Autodesk Inventor part; units mm, degrees
ref_plane "YZ Plane" through (0, 0, 0) normal (1, 0, 0) x (0, 1, 0)
ref_plane "XZ Plane" through (0, 0, 0) normal (0, 1, 0) x (-1, 0, 0)
ref_plane "XY Plane" through (0, 0, 0) normal (0, 0, 1) x (1, 0, 0)
sketch "Sketch1" plane through (0, 0, 0) normal (0, 1, 0) x (-1, 0, 0)
  line L0 (26, 37.5) -> (-26, 37.5)
  line L1 (-26, 37.5) -> (-26, -37.5)
  line L2 (-26, -37.5) -> (26, -37.5)
  line L3 (26, -37.5) -> (26, 37.5)
  line L4 (26, 37.5) -> (-26, -37.5) construction
  line L5 (-26, 37.5) -> (26, -37.5) construction
  point P0 (0, 0)
  dimension "d0" = 52
  dimension "d1" = 75
extrude "Extrusion1" add sketch "Sketch1" along normal blind 5
sketch "Sketch2" plane through (0, 5, 0) normal (0, 1, 0) x (1, 0, 0)
  line L0 (-13, -33.5) -> (35.879, -33.5)
  line L1 (-26, -37.5) -> (26, -37.5)
  line L2 (-23, -23.5) -> (-23, 74.0013)
  line L3 (-26, 37.5) -> (-26, -37.5)
  arc A0 (-23, 23.5) -> (-13, 33.5) centre (-23, 33.5) ccw
  line L4 (26, 37.5) -> (-26, 37.5)
  arc A1 (13, 33.5) -> (23, 23.5) centre (23, 33.5) ccw
  line L5 (26, -37.5) -> (26, 37.5)
  line L6 (-13, 33.5) -> (13, 33.5)
  line L7 (18, -33.5) -> (23, 23.5)
  arc A2 (-23, -23.5) -> (-13, -33.5) centre (-13, -23.5) ccw
  point P0 (0, 0)
  dimension "d4" = 4
  dimension "d5" = 3
  dimension "d6" = 20
  dimension "d7" = 4
  dimension "d8" = 20
  dimension "d9" = 4
  dimension "d10" = 3
  dimension "d11" = 8
  dimension "d12" = 3
  dimension "d13" = 10
extrude "Extrusion2" add sketch "Sketch2" along normal blind 3 contours A2 L2 A0 L6 A1 L7 L0
sketch "Sketch3" plane through (0, 8, 0) normal (0, 1, 0) x (1, 0, 0)
  line L0 (4, -10.5) -> (4, -24.5)
  line L1 (7, -27.5) -> (13, -27.5)
  line L2 (16, -24.5) -> (16, -10.5)
  line L3 (13, -7.5) -> (7, -7.5)
  line L4 (26, -37.5) -> (26, 37.5)
  line L5 (-26, -37.5) -> (26, -37.5)
  arc A0 (4, -24.5) -> (7, -27.5) centre (7, -24.5) ccw
  arc A1 (7, -7.5) -> (4, -10.5) centre (7, -10.5) ccw
  arc A2 (16, -10.5) -> (13, -7.5) centre (13, -10.5) ccw
  arc A3 (13, -27.5) -> (16, -24.5) centre (13, -24.5) ccw
  arc A4 (-9, -23.5) -> (-9, -29.5) centre (-9, -26.5) ccw
  arc A5 (-1, -29.5) -> (-1, -23.5) centre (-1, -26.5) ccw
  line L6 (-9, -23.5) -> (-1, -23.5)
  line L7 (-9, -29.5) -> (-1, -29.5)
  circle A6 centre (0, 13.5) radius 7.5
  circle A7 centre (0, 2) radius 3
  circle A8 centre (-8.1317, 5.3683) radius 3
  circle A9 centre (-11.5, 13.5) radius 3
  circle A10 centre (-8.1317, 21.6317) radius 3
  circle A11 centre (0, 25) radius 3
  circle A12 centre (8.1317, 21.6317) radius 3
  circle A13 centre (11.5, 13.5) radius 3
  circle A14 centre (8.1317, 5.3683) radius 3
  point P0 (0, 0)
  point P1 (4, -7.5)
  point P2 (4, -27.5)
  point P3 (16, -27.5)
  dimension "d16" = 22
  dimension "d17" = 30
  dimension "d18" = 20
  dimension "d19" = 12
  dimension "d20" = 3
  dimension "d21" = 6
  dimension "d22" = 6
  dimension "d23" = 27
  dimension "d24" = 11
  dimension "d25" = 11
  dimension "d26" = 35
  dimension "d27" = 15
  dimension "d28" = 51
  dimension "d29" = 26
  dimension "d30" = 6
  dimension "d31" = 11.5
  dimension "d34" = 360
extrude "Extrusion3" cut sketch "Sketch3" against normal blind 4 contours A1 L3 A2 L2 A3 L1 A0 L0 | L6 A5 L7 A4 | A7 | A8 | A9 | A10 | A11 | A12 | A13 | A14
sketch "Sketch4" plane through (0, 8, 0) normal (0, 1, 0) x (1, 0, 0)
  circle A0 centre (0, 13.5) radius 7.5
  line L0 (26, -37.5) -> (26, 37.5)
  line L1 (-26, -37.5) -> (26, -37.5)
  circle A1 centre (0, 13.5) radius 15.5
  point P0 (0, 0)
  dimension "d38" = 15
  dimension "d39" = 26
  dimension "d40" = 51
  dimension "d41" = 31
extrude "Extrusion4" cut sketch "Sketch4" against normal blind 2
properties part number "A2P2"
Read the model definition and answer for the solid it produces. Units are mm, in the model's axes. A direction names the side the tool comes from. Round coordinates to 2 decimals unless told otherwise and drop trailing zeros. Write each loop counter-clockwise with the first axis right and the second up, starting at its lowest first coordinate (ties: lowest second). Pieces come first, ordered by that corner, then holes.
1. Determine the mould class of faces 1 (the face through (-12, 4, -14)), 2 (the face through (16.01, 6.48, -26.35)), 3 (the face through (20.465, 6.479, 5.399)) for opening direction Z: pulls with the +Z half, pulls with the -Z half, needs draft (parallel to the pull), parting line crosses it, or undercut.
2. The part is cut by section D-D, the plane x = 21.5. Determine the outline of the cut face in (y, z).
3. The part is cut by section C-C, the plane z = -13.5. Determine the outline of the cut face in (x, y), then the cut area to 3 significant figures.
4. The part is cut by section A-A, the plane x = -2. Determine the outline of the cut face in (y, z), then the cut area to 3 significant figures.
5. Given pin 1 Ø7 at (x, z) = (11.5, -13.5) entering from +Y; pin 2 Ø5 at (x, z) = (8.13, -5.37) entering from +Y, each flat-ended and moving along its own axis, determine where each tip first touches the part or whether it passes through.
6. The part is cut by section B-B, the plane z = 26.5. Determine the outline of the cut face in (x, y).
7. Straight lines are drawn through the part: L1, parallel to Z at x = 11.5, y = 5.15; L2, parallel to X at y = 7.5, z = -13.5; L3, parallel to X at y = 6.5, z = -17. For each, find the intervals that lie inside material, in ascending order.
8. Which of the six approach directions +Z, -Z, +X, -X, +Y, -Y give full straight-line access (tool end or side, diameter ignored) to faces 4 (the face through (-15.85, 6.48, -26.51)), 5 (the face through (-5, 6, 29.5)), 6 (the face through (-26, 2, -1))?
Values:
1. face 1: undercut
1. face 2: pulls with the -Z half
1. face 3: pulls with the +Z half
2. outline: (0, -37.5) - (5, -37.5) - (5, -23.61) - (8, -23.61) - (8, -6.4) - (5, -6.4) - (5, 37.5) - (0, 37.5) - close
3. outline: (-26, 0) - (26, 0) - (26, 5) - (22.12, 5) - (22.12, 8) - (15.5, 8) - (15.5, 6) - (14.5, 6) - (14.5, 4) - (8.5, 4) - (8.5, 6) - (7.5, 6) - (7.5, 8) - (-7.5, 8) - (-7.5, 6) - (-8.5, 6) - (-8.5, 4) - (-14.5, 4) - (-14.5, 6) - (-15.5, 6) - (-15.5, 8) - (-23, 8) - (-23, 5) - (-26, 5) - close
3. area: 339 mm2
4. outline: (0, -37.5) - (5, -37.5) - (5, -33.5) - (8, -33.5) - (8, -28.87) - (6, -28.87) - (6, -27.24) - (4, -27.24) - (4, -22.76) - (6, -22.76) - (6, -20.73) - (8, -20.73) - (8, -6.27) - (6, -6.27) - (6, -4.24) - (4, -4.24) - (4, 0.24) - (6, 0.24) - (6, 1.87) - (8, 1.87) - (8, 23.5) - (4, 23.5) - (4, 29.5) - (8, 29.5) - (8, 33.5) - (5, 33.5) - (5, 37.5) - (0, 37.5) - close
4. area: 502 mm2
5. pin 1: stops at y = 6
5. pin 2: stops at y = 4
6. outline: (-26, 0) - (26, 0) - (26, 5) - (18.61, 5) - (18.61, 8) - (15.24, 8) - (15.24, 4) - (4.76, 4) - (4.76, 8) - (2, 8) - (2, 4) - (-12, 4) - (-12, 8) - (-22.54, 8) - (-22.54, 5) - (-26, 5) - close
7. L1: z = -33.5 to -16.5, -10.5 to 7.5, 27.5 to 33.5
7. L2: x = -23 to -15.5, -7.5 to 7.5, 15.5 to 22.12
7. L3: x = -23 to -15.1, -6.63 to 6.63, 15.1 to 22.43
8. face 4: -Z, -X, +Y
8. face 5: +Y
8. face 6: +Z, -Z, -X, +Y, -Y
